from build123d import *

# Parameters (mm, degrees)
SKETCH_1_R          = 1.5
EXTRUDE_1_DEPTH     = 8
EXTRUDE_2_DEPTH     = 4
SKETCH_4_W          = 7
SKETCH_4_H          = 14
EXTRUDE_3_DEPTH     = 10
CUT_EXTRUDE_START   = -3
CUT_EXTRUDE_1_DEPTH = 7
SKETCH_6_W          = 7
SKETCH_6_H          = 5.039650546
CUT_EXTRUDE_3_DEPTH = 10
CUT_EXTRUDE_START_2 = -10
SKETCH_7_R          = 1.5
CUT_EXTRUDE_4_DEPTH = 10
SKETCH_9_W          = 8
SKETCH_9_H          = 3
EXTRUDE_4_DEPTH     = 7
FILLET_3_R          = 3
FILLET_4_R          = 2
SKETCH_10_W         = 4
SKETCH_10_H         = 4
EXTRUDE_5_DEPTH     = 10
SKETCH_8_R          = 2
CUT_EXTRUDE_6_DEPTH = 10
SKETCH_13_R         = 2.5
CUT_EXTRUDE_7_DEPTH = 1
SKETCH_14_W         = 8
SKETCH_14_H         = 3
EXTRUDE_6_DEPTH     = 7
FILLET_5_R          = 2
SKETCH_15_R         = 2
CUT_EXTRUDE_8_DEPTH = 7


with BuildPart() as part:
    # 草图1 → 凸台-拉伸1 (new body)
    with BuildSketch(Plane.XY):
        Polygon((16, 7), (-16, 7), (-16, -7), (-12, -7), (-12, 4), (12, 4), (12, -7), (16, -7), align=None)
        with Locations((-14, -3)):
            Circle(SKETCH_1_R, mode=Mode.SUBTRACT)
        with Locations((14, -3)):
            Circle(SKETCH_1_R, mode=Mode.SUBTRACT)
    extrude(amount=EXTRUDE_1_DEPTH)

    # 草图3 → 凸台-拉伸2 (add)
    with BuildSketch(Plane(origin=(0, 0, 0), x_dir=(-1, 0, 0), z_dir=(0, 0, -1))):
        with BuildLine():
            Line((2, -7), (12, -7))
            Line((12, -7), (12, 1.960349454))
            Line((12, 1.960349454), (2, 1.960349454))
            Line((2, 1.960349454), (2, 0))
            ThreePointArc((2, 0), (4.121320344, -0.878679656), (5, -3))
            ThreePointArc((5, -3), (4.121320344, -5.121320344), (2, -6))
            Line((2, -6), (2, -7))
        make_face()
    extrude(amount=-EXTRUDE_2_DEPTH)

    # 草图4 → 凸台-拉伸3 (add)
    with BuildSketch(Plane(origin=(0, 0, 0), x_dir=(-1, 0, 0), z_dir=(0, 0, -1))):
        with Locations((12.5, 0)):
            Rectangle(SKETCH_4_W, SKETCH_4_H)
    extrude(amount=EXTRUDE_3_DEPTH)

    # 草图5 → 切除-拉伸1 (cut)
    with BuildSketch(Plane(origin=(0, 0, -10), x_dir=(-1, 0, 0), z_dir=(0, 0, -1)).offset(CUT_EXTRUDE_START)):
        with BuildLine():
            ThreePointArc((12.209881979, -3), (11.697318846, -1.762563133), (10.459881979, -1.25))
            ThreePointArc((10.459881979, -1.25), (9.631108119, -1.458690852), (9, -2.034989841))
            Line((9, -2.034989841), (9, -3.965010159))
            ThreePointArc((9, -3.965010159), (10.963720513, -4.675901767), (12.209881979, -3))
        make_face()
        with BuildLine():
            Line((9, -3.965010159), (9, -2.034989841))
            ThreePointArc((9, -2.034989841), (8.709881979, -3), (9, -3.965010159))
        make_face()
        with BuildLine():
            ThreePointArc((11.753305584, -7), (12.095368491, -5.012986712), (12.209881979, -3))
            ThreePointArc((12.209881979, -3), (10.963720513, -4.675901767), (9, -3.965010159))
            Line((9, -3.965010159), (9, -7))
            Line((9, -7), (11.753305584, -7))
        make_face()
        with BuildLine():
            Line((10.459881979, -1.25), (9, -1.204378688))
            Line((9, -1.204378688), (9, -2.034989841))
            ThreePointArc((9, -2.034989841), (9.631108119, -1.458690852), (10.459881979, -1.25))
        make_face()
    extrude(amount=-CUT_EXTRUDE_1_DEPTH, mode=Mode.SUBTRACT)

    # 草图6 → 切除-拉伸3 (cut)
    with BuildSketch(Plane(origin=(0, 0, -10), x_dir=(-1, 0, 0), z_dir=(0, 0, -1))):
        with Locations((12.5, 4.480174727)):
            Rectangle(SKETCH_6_W, SKETCH_6_H)
    extrude(amount=-CUT_EXTRUDE_3_DEPTH, mode=Mode.SUBTRACT)

    # 草图7 → 切除-拉伸4 (cut)
    with BuildSketch(Plane.XY.offset(CUT_EXTRUDE_START_2)):
        with Locations((-14, -3)):
            Circle(SKETCH_7_R)
    extrude(amount=CUT_EXTRUDE_4_DEPTH, mode=Mode.SUBTRACT)

    # 草图9 → 凸台-拉伸4 (add)
    with BuildSketch(Plane(origin=(16, 0, 0), x_dir=(0, 0, -1), z_dir=(1, 0, 0))):
        with Locations((-4, 5.5)):
            Rectangle(SKETCH_9_W, SKETCH_9_H)
    extrude(amount=EXTRUDE_4_DEPTH)

    # 圆角3
    # the kernel refuses this fillet: 3 mm, written as the material it adds along each edge
    with BuildSketch(Plane(origin=(-16, 1.960349454, 0), x_dir=(0, 0, -1), z_dir=(1, 0, 0))) as fillet_3_piece_1:
        with BuildLine():
            CenterArc((FILLET_3_R, FILLET_3_R), FILLET_3_R, 180, 90)
            Line((0, FILLET_3_R), (0, 0))
            Line((0, 0), (FILLET_3_R, 0))
        make_face()
    extrude(amount=4)
    with BuildSketch(Plane(origin=(16, 4, 0), x_dir=(1, 0, 0), z_dir=(0, 0, 1))) as fillet_3_piece_2:
        with BuildLine():
            CenterArc((FILLET_3_R, -FILLET_3_R), FILLET_3_R, 90, 90)
            Line((0, -FILLET_3_R), (0, 0))
            Line((0, 0), (FILLET_3_R, 0))
        make_face()
    extrude(amount=8)

    # 圆角4
    fillet_4_edges = [part.edges().sort_by_distance(p)[0] for p in [
        (-12, 4, 4),
    ]]
    fillet(fillet_4_edges, radius=FILLET_4_R)

    # 草图10 → 凸台-拉伸5 (add)
    with BuildSketch(Plane.XZ.offset(7)):
        with Locations((14, 6)):
            Rectangle(SKETCH_10_W, SKETCH_10_H)
    extrude(amount=EXTRUDE_5_DEPTH)

    # 草图8 → 切除-拉伸6 (cut)
    with BuildSketch(Plane(origin=(0, 7, 0), x_dir=(1, 0, 0), z_dir=(0, 1, 0))):
        with Locations(Location((7, -4, 0), (0, 0, 270))):
            Circle(SKETCH_8_R)
        with Locations((27, -4)):
            Circle(SKETCH_8_R)
    extrude(amount=-CUT_EXTRUDE_6_DEPTH, mode=Mode.SUBTRACT)

    # 草图13 → 切除-拉伸7 (cut)
    with BuildSketch(Plane.XZ.offset(-4)):
        with Locations(Location((7, 4, 0), (0, 0, 270))):
            Circle(SKETCH_13_R)
    extrude(amount=-CUT_EXTRUDE_7_DEPTH, mode=Mode.SUBTRACT)

    # 草图14 → 凸台-拉伸6 (add)
    with BuildSketch(Plane(origin=(23, 0, 0), x_dir=(0, 0, -1), z_dir=(1, 0, 0))):
        with Locations((-4, 5.5)):
            Rectangle(SKETCH_14_W, SKETCH_14_H)
    extrude(amount=EXTRUDE_6_DEPTH)

    # 圆角5
    fillet_5_edges = [part.edges().sort_by_distance(p)[0] for p in [
        (12, 4, 4),
    ]]
    fillet(fillet_5_edges, radius=FILLET_5_R)

    # 草图15 → 切除-拉伸8 (cut)
    with BuildSketch(Plane(origin=(0, 7, 0), x_dir=(1, 0, 0), z_dir=(0, 1, 0))):
        with Locations(Location((27, -4, 0), (0, 0, 270))):
            Circle(SKETCH_15_R)
        with Locations(Location((7, -4, 0), (0, 0, 270))):
            Circle(SKETCH_15_R)
    extrude(amount=-CUT_EXTRUDE_8_DEPTH, mode=Mode.SUBTRACT)


solid = part.part
Build history of the part. All positions in model axes, mm. A direction names the side the tool comes from. Round coordinates to 2 decimals unless told otherwise and drop trailing zeros. Write each loop counter-clockwise with the first axis right and the second up, starting at its lowest first coordinate (ties: lowest second). Pieces come first, ordered by that corner, then holes. Notation, with made-up numbers: (11.25, 18) - (51.25, 18) arc R19 cw to (51.25, 22) - close; hole circle Ø2 at (20, -24.5). An arc over 180 degrees is marked (long way). Use CSV: the item, a comma, the result in double quotes.
(1) Band-saw the part on D-D (z = -8.25). Write the cut outline in (x, y).
Response:
outline,"(-16, -7) - (-9, -7) - (-9, 1.96) - (-16, 1.96) - close; hole circle Ø3 at (-14, -3)"
(2) Wall check: line 1 (Y direction, x = -6.5, z = 2); line 2 (Y direction, x = -14, z = -3); line 3 (X direction, y = -1.75, z = 3). Give the ranges that are in metal, low to high.
Response:
line 1,"-7 to 1.96, 4 to 7"
line 2,"-7 to -4.5, -1.5 to 1.96"
line 3,"-16 to -14.83, -13.17 to -4.73, 12 to 13.17, 14.83 to 16"
(3) Band-saw the part on B-B (x = -14). Write the cut outline in (y, z), plus the area to 3 significant figures.
Response:
outline,"(-7, -10) - (-4.5, -10) - (-4.5, 8) - (-7, 8) - close; (-1.5, -10) - (1.96, -10) - (1.96, -3) arc R3 cw to (4.96, 0) - (7, 0) - (7, 8) - (-1.5, 8) - close"
area,"150 mm²"
(4) Band-saw the part on C-C (y = -2.5). Write the cut outline in (x, z).
Response:
outline,"(-16, -10) - (-15.41, -10) - (-15.41, 8) - (-16, 8) - close; (-12.59, -10) - (-9, -10) - (-9, -7) - (-12.14, -7) - (-12.14, 0) - (-4.96, 0) - (-4.96, 4) - (-12, 4) - (-12, 8) - (-12.59, 8) - close; (12, 0) - (12.59, 0) - (12.59, 8) - (12, 8) - close; (15.41, 0) - (16, 0) - (16, 8) - (15.41, 8) - close"
(5) 3-axis set-ups, long thin cutter, end or side, ignore diameter. For faces 1 (the flat face through (-12, -7, -1)), 2 (the flat face through (-12, -2, -10)), 3 (the flat face through (9, 5, 5)), 4 (the flat face through (24, 4, 4)), 5 (the flat face through (-8, -2, 4)): which of +Z, -Z, +X, -X, +Y, -Y reach the whole face in a straight line?
Response:
face 1,"+Z, -Z, -X, -Y"
face 2,"-Z, +X, -X, +Y, -Y"
face 3,"-Y"
face 4,"+Z, -Z, +X, -Y"
face 5,"+Z, -Y"
(6) Mould opens along Y. For faces 6 (the cylindrical face through (-15.5, -2.93, -1.13)), 7 (the flat face through (14, -7, 2)), 8 (the flat face through (-2, 1, 2)), 9 (the cylindrical face through (-11.4, 3.43, 4.06)) say: pulls with the +Y half, pulls with the -Y half, needs draft (parallel to the pull), parting line crosses it, or undercut.
Response:
face 6,"undercut"
face 7,"pulls with the -Y half"
face 8,"needs draft"
face 9,"undercut"
(7) Band-saw the part on A-A (z = 2.5). Give the number of separate pieces and of enclosed holes in the cut face, plus the area to 3 significant figures.
Response:
separate pieces,"3"
enclosed holes,"2"
area,"274 mm²"
(8) Pin check, flat tips, straight feed: P1, Ø1.5, axis at x = -7.5, y = -3, coming from the -Z side; P2, Ø4.5, axis at y = -4, z = -4, coming from the +X side; P3, Ø0.5, axis at y = -6.5, z = 1, coming from the +X side. Stop position of each tip, or through.
Response:
P1,"z = 0"
P2,"x = -11.68"
P3,"x = 16"
